```python
from build123d import *

# Parameters (mm, degrees)
CROQUIS1_W              = 18
CROQUIS1_H              = 80
SALIENTE_EXTRUIR1_DEPTH = 50
CROQUIS2_W              = 16
CROQUIS2_H              = 18
CORTAR_EXTRUIR1_DEPTH   = 25
SALIENTE_EXTRUIR2_DEPTH = 18
CROQUIS4_W              = 6.99659876
CROQUIS4_H              = 2.653687506
SALIENTE_EXTRUIR3_DEPTH = 2
CORTAR_EXTRUIR2_DEPTH   = 6.996599
CROQUIS6_W              = 6.99659876
CROQUIS6_H              = 3.5
SALIENTE_EXTRUIR4_DEPTH = 6
CROQUIS7_W              = 16.864509826
CROQUIS7_H              = 3.5
SALIENTE_EXTRUIR5_DEPTH = 4
CROQUIS8_R              = 4
CORTAR_EXTRUIR3_DEPTH   = 3


with BuildPart() as part:
    # Croquis1 → Saliente-Extruir1 (new body)
    with BuildSketch(Plane.XY):
        with Locations((9, -40)):
            Rectangle(CROQUIS1_W, CROQUIS1_H)
    extrude(amount=-SALIENTE_EXTRUIR1_DEPTH)

    # Croquis2 → Cortar-Extruir1 (cut)
    with BuildSketch(Plane.ZY):
        with Locations((-8, -9)):
            Rectangle(CROQUIS2_W, CROQUIS2_H)
        with Locations((-8, -71)):
            Rectangle(CROQUIS2_W, CROQUIS2_H)
    extrude(amount=-CORTAR_EXTRUIR1_DEPTH, mode=Mode.SUBTRACT)

    # Croquis3 → Saliente-Extruir2 (add)
    with BuildSketch(Plane.ZY):
        with BuildLine():
            Line((0, -33.158339238), (0, -46.786065604))
            ThreePointArc((0, -46.786065604), (1.471610076, -43.53202647), (2, -40))
            ThreePointArc((2, -40), (1.417568162, -36.457103303), (0, -33.158339238))
        make_face()
    extrude(amount=-SALIENTE_EXTRUIR2_DEPTH)

    # Croquis4 → Saliente-Extruir3 (add)
    with BuildSketch(Plane.XY):
        with Locations((9, -36.579169619)):
            Rectangle(CROQUIS4_W, CROQUIS4_H)
    extrude(amount=SALIENTE_EXTRUIR3_DEPTH)

    # Croquis5 → Cortar-Extruir2 (cut)
    with BuildSketch(Plane.ZY.offset(-5.50170062)):
        Polygon((2, -37.906013372), (-1.355869072, -36.911959665), (-0.421934466, -33.759049274), (2.933934606, -34.75310298), align=None)
    extrude(amount=-CORTAR_EXTRUIR2_DEPTH, mode=Mode.SUBTRACT)

    # Croquis6 → Saliente-Extruir4 (add)
    with BuildSketch(Plane(origin=(0, -34.303696532, -10.16121784), x_dir=(1, 0, 0), z_dir=(0, 0.958819735, 0.284015345))):
        with Locations((9, -10.933528924)):
            Rectangle(CROQUIS6_W, CROQUIS6_H)
    extrude(amount=SALIENTE_EXTRUIR4_DEPTH)

    # Croquis7 → Saliente-Extruir5 (add)
    with BuildSketch(Plane(origin=(0, -28.550778123, -8.457125772), x_dir=(1, 0, 0), z_dir=(0, 0.958819735, 0.284015345))):
        with Locations((9, -10.933528924)):
            Rectangle(CROQUIS7_W, CROQUIS7_H)
    extrude(amount=SALIENTE_EXTRUIR5_DEPTH)

    # Croquis8 → Cortar-Extruir3 (cut)
    with BuildSketch(Plane.XY.offset(-16)):
        with Locations((9, -9)):
            Circle(CROQUIS8_R)
        with Locations((9, -71)):
            Circle(CROQUIS8_R)
    extrude(amount=-CORTAR_EXTRUIR3_DEPTH, mode=Mode.SUBTRACT)


solid = part.part
```
Check sheet for the modelled part. Datum: model origin and axes. Units: mm. A direction names the side the tool comes from. Round coordinates to 2 decimals unless told otherwise and drop trailing zeros. Order: outer loops, then holes, each group sorted by start corner. A loop starts at its lowest first (then second) coordinate and runs counter-clockwise, first axis right, second up.
1) Mould release check, pull along X, two halves, no side actions. Record for faces 1 (the flat face through (17.432, -30, 3)), 2 (the flat face through (9, -54, 0)), 3 (the flat face through (9, -71, -19)), 4 (the flat face through (0, -41, -29)): +X half, -X half, draft (parallel to the pull), parting line (faces both ways), or undercut.
2) Tool access check on faces 5 (the flat face through (14.93, -31.65, 2)), 6 (the flat face through (9, -18, -8)), 7 (the flat face through (9, -62, -8)), 8 (the cylindrical face through (8.133, -74.905, -17.479)), 9 (the flat face through (3, -31.65, 2)). Record the directions out of +Z, -Z, +X, -X, +Y, -Y that give a thin tool (end or side, any length) a straight path to the whole face; none if there is none.
3) Section check A-A (x = 16). Record the boundary of the cut face in (y, z), and give its area (3 significant figures).
4) Go/stop test with flat-tipped pins: pin 1 Ø5 at (x, z) = (15.5, -3.5) entering from -Y; pin 2 Ø6.5 at (x, y) = (7, -71) entering from +Z; pin 3 Ø1.3 at (y, z) = (-30.5, 3) entering from +X. Record where each tip stops, or that it passes through.
5) Section check C-C (x = 9). Record the boundary of the cut face in (y, z).
6) Section check B-B (z = -17). Record the boundary of the cut face in (x, y).
7) Scan lines: line 1 (Y direction, x = 9, z = -18.3); line 2 (Z direction, x = 5, y = -3.5); line 3 (Z direction, x = 7.75, y = -23). Record each from-to range of solid material in increasing order.
8) Section check D-D (y = -9). Record the boundary of the cut face in (x, z).
Result:
1. face 1: +X half
1. face 2: draft
1. face 3: undercut
1. face 4: -X half
2. face 5: +X
2. face 6: +Z, +X, -X, +Y
2. face 7: +Z, +X, -X, -Y
2. face 8: +Z
2. face 9: -X
3. outline: (-80, -50) - (0, -50) - (0, -16) - (-18, -16) - (-18, 0) - (-33.16, 0) arc R14.82 ccw to (-40, 2) arc R12.97 ccw to (-46.79, 0) - (-62, 0) - (-62, -16) - (-80, -16) - close; (-32.15, 3.7) - (-31.16, 0.35) - (-27.32, 1.48) - (-28.32, 4.84) - close
3. area: 3,460 mm2
4. pin 1: stops at y = -62
4. pin 2: stops at z = -16
4. pin 3: stops at x = 17.43
5. outline: (-80, -50) - (0, -50) - (0, -16) - (-5, -16) - (-5, -19) - (-13, -19) - (-13, -16) - (-18, -16) - (-18, 0) - (-32.33, 0) - (-27.32, 1.48) - (-28.32, 4.84) - (-37.91, 2) - (-37.91, 1.76) arc R14.82 ccw to (-40, 2) arc R12.97 ccw to (-46.79, 0) - (-62, 0) - (-62, -16) - (-67, -16) - (-67, -19) - (-75, -19) - (-75, -16) - (-80, -16) - close
6. outline: (0, -80) - (18, -80) - (18, 0) - (0, 0) - close; hole circle Ø8 at (9, -71); hole circle Ø8 at (9, -9)
7. line 1: y = -80 to -75, -67 to -13, -5 to 0
7. line 2: z = -50 to -16
7. line 3: z = -50 to 0
8. outline: (0, -50) - (18, -50) - (18, -16) - (13, -16) - (13, -19) - (5, -19) - (5, -16) - (0, -16) - close
